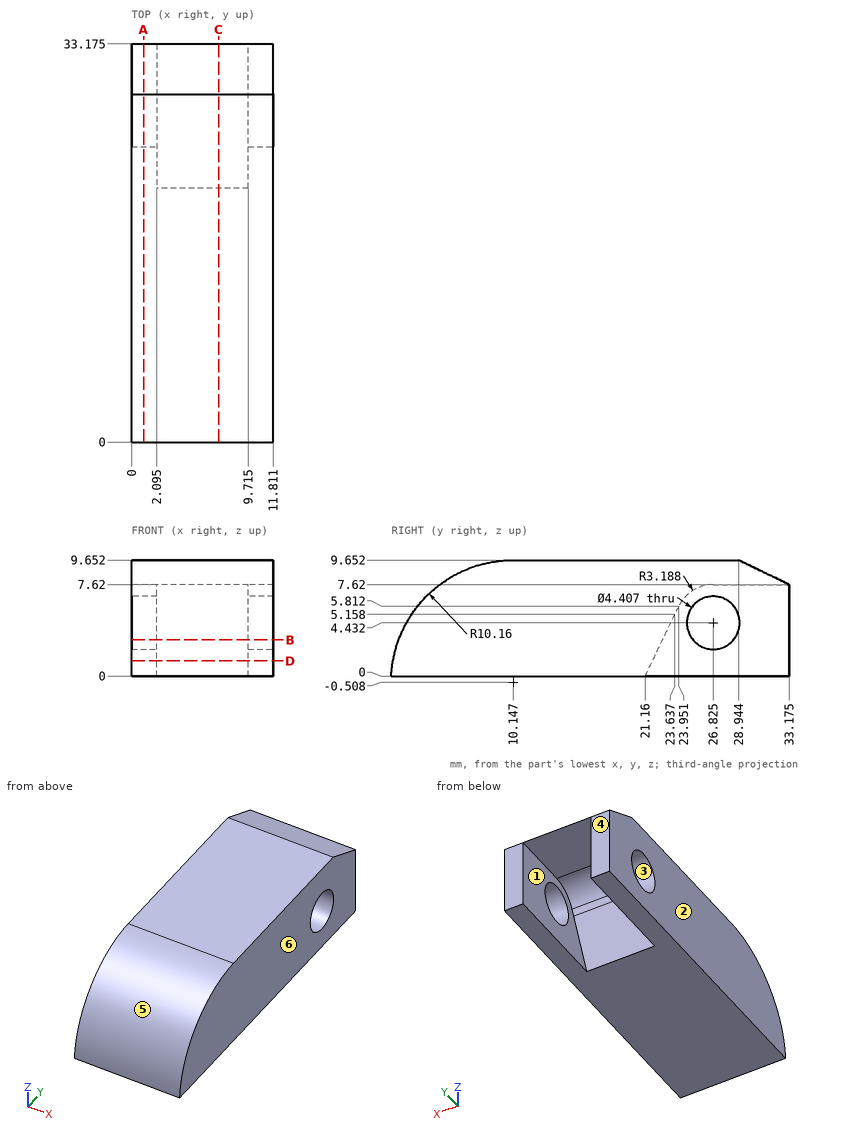
Geometry: see drawing. Coordinates: mm, zero at the bounding-box minimum. A direction names the side the tool comes from. Coordinates: 2 decimals unless noted, no trailing zeros. Write each loop counter-clockwise with the first axis right and the second up, starting at its lowest first coordinate (ties: lowest second). Pieces come first, ordered by that corner, then holes.
1) Mould query, pull axis Y, two halves, no side actions, for the marked faces 3, 4, 5 and 6. Classes: pulls with the +Y half, pulls with the -Y half, needs draft (parallel to the pull), parting line crosses it, or undercut.
2) Section A-A on x = 1. Output: boundary loops of the cut face in (y, z) (1 decimal), and give its area (3 significant figures).
3) Material intervals for line 1 along X through (y, z) = (24, 3.5) (1 decimal); line 2 along Y through (x, z) = (10, 6.25) (1 decimal); line 3 along Z through (x, y) = (7.5, 27.5), sorted ascending.
4) Section B-B on z = 3. State how many separate pieces and enclosed holes the cut face has, and give its area (3 significant figures).
5) Section D-D on z = 1.25. Output: boundary loops of the cut face in (x, y) (1 decimal).
6) Pin query (flat end, axial travel): pin 1 Ø1.5 at (x, z) = (1.5, 6) entering from -Y (1 decimal); pin 2 Ø3 at (x, z) = (4.5, 3) entering from +Y; pin 3 Ø1.5 at (x, y) = (6, 23.5) entering from -Z. Return the tip coordinate at first contact, or that it passes through.
7) Section C-C on x = 7.25. Output: boundary loops of the cut face in (y, z) (1 decimal).
8) Set-up query: the marked faces 1 and 2. Return all of +Z, -Z, +X, -X, +Y, -Y with unobstructed straight access to the full face (end or side cutting, diameter ignored); none if empty.
Check result:
1. face 3: undercut
1. face 4: pulls with the +Y half
1. face 5: pulls with the -Y half
1. face 6: needs draft
2. outline: (0, 0) - (33.2, 0) - (33.2, 7.6) - (28.9, 9.7) - (10.1, 9.7) arc R10.2 ccw to start; hole circle Ø4.4 at (26.8, 4.4)
2. area: 279 mm2
3. line 1: x = 0 to 2.1, 9.7 to 11.8
3. line 2: y = 2.6 to 25.6, 28.1 to 33.2
3. line 3: z = 7.62 to 9.65
4. separate pieces: 3
4. enclosed holes: 0
4. area: 290 mm2
5. outline: (0, 0.1) - (11.8, 0.1) - (11.8, 33.2) - (9.7, 33.2) - (9.7, 21.8) - (2.1, 21.8) - (2.1, 33.2) - (0, 33.2) - close
6. pin 1: stops at y = 1.8
6. pin 2: stops at y = 23.32
6. pin 3: stops at z = 3.31
7. outline: (0, 0) - (21.2, 0) - (24, 5.8) arc R3.2 cw to (26.8, 7.6) - (33.2, 7.6) - (28.9, 9.7) - (10.1, 9.7) arc R10.2 ccw to start
8. face 1: -Z, +Y
8. face 2: +Z, -Z, -X, +Y, -Y
